```python
from build123d import *

# Parameters (mm, degrees)
EXTRUDE_1_DEPTH     = 12
SKETCH_2_R          = 8
CUT_EXTRUDE_1_DEPTH = 8
SKETCH_3_R          = 2.5
CUT_EXTRUDE_2_DEPTH = 10


with BuildPart() as part:
    # 草图1 → 凸台-拉伸1 (new body)
    with BuildSketch(Plane(origin=(0, 0, 0), x_dir=(0, 0, -1), z_dir=(1, 0, 0))):
        with BuildLine():
            Line((-27, 20), (27, 20))
            ThreePointArc((27, 20), (30.535533906, 18.535533906), (32, 15))
            Line((32, 15), (32, -15))
            ThreePointArc((32, -15), (30.535533906, -18.535533906), (27, -20))
            Line((27, -20), (-27, -20))
            ThreePointArc((-27, -20), (-30.535533906, -18.535533906), (-32, -15))
            Line((-32, -15), (-32, 15))
            ThreePointArc((-32, 15), (-30.535533906, 18.535533906), (-27, 20))
        make_face()
    extrude(amount=EXTRUDE_1_DEPTH)

    # 草图2 → 切除-拉伸1 (cut)
    with BuildSketch(Plane.ZY):
        Circle(SKETCH_2_R)
    extrude(amount=-CUT_EXTRUDE_1_DEPTH, mode=Mode.SUBTRACT)

    # 草图3 → 切除-拉伸2 (cut)
    with BuildSketch(Plane.XZ.offset(20)):
        with Locations((4, 0)):
            Circle(SKETCH_3_R)
    extrude(amount=-CUT_EXTRUDE_2_DEPTH, mode=Mode.SUBTRACT)


solid = part.part
```
Here's how the part is built. I have some questions about the finished solid (model axes, mm). A direction names the side the tool comes from. Coordinates: 2 decimals unless noted, no trailing zeros. Write each loop counter-clockwise with the first axis right and the second up, starting at its lowest first coordinate (ties: lowest second). Pieces come first, ordered by that corner, then holes. Notation, with made-up numbers: (-33.5, 64.5) -> (-15.5, 64.5) arc R16 cw to (-15.5, 80.5) -> close; hole circle Ø8 at (1, 16). An arc over 180 degrees is marked (long way). Use a Markdown table: item, result. Add a question column.
(1) If we section it at C-C, the plane z = 0: Write out the boundary of the cut face in (x, y), and give its area (3 significant figures).
(2) If we section it at B-B, the plane y = 0: Write out the boundary of the cut face in (x, z), and give its area (3 significant figures).
(3) For faces 1 (the flat face through (7, -20, 0)), 2 (the flat face through (8, 0, 0)), 3 (the cylindrical face through (6.385, -15.07, 0.751)), which set-ups out of +Z, -Z, +X, -X, +Y, -Y let a thin tool reach every point of the face, with its end or its side?
(4) I'm going to push flat-ended pins straight in: P1, Ø1.5, axis at x = 4, z = 0.5, coming from the -Y side; P2, Ø5, axis at y = 0.5, z = -0.5, coming from the -X side. Where does each tip first touch, or does it pass through?
(5) Please list where these lines run through material, in increasing order: line 1 (Y direction, x = 5.75, z = 0); line 2 (Z direction, x = 7.5, y = 1); line 3 (Z direction, x = 4, y = -18).
(6) If we section it at D-D, the plane y = -5.5: Write out the boundary of the cut face in (x, z).
(7) We'd pull the mould along X, two halves only. Please class faces 4 (the cylindrical face through (6, 19, -30)), 5 (the flat face through (12, 0, 0)), 6 (the flat face through (0, 5, -8)), 7 (the flat face through (4, -10, 0)): +X half, -X half, draft (parallel to the pull), parting line (faces both ways), or undercut.
(8) If we section it at A-A, the plane x = 4: Write out the boundary of the cut face in (y, z), and give its area (3 significant figures).
Outcome:
| question | item | result |
|---|---|---|
| 1 | outline | (0, -20) -> (1.5, -20) -> (1.5, -10) -> (6.5, -10) -> (6.5, -20) -> (12, -20) -> (12, 20) -> (0, 20) -> (0, 8) -> (8, 8) -> (8, -8) -> (0, -8) -> close |
| 1 | area | 302 mm^2 |
| 2 | outline | (0, -32) -> (12, -32) -> (12, 32) -> (0, 32) -> (0, 8) -> (8, 8) -> (8, -8) -> (0, -8) -> close |
| 2 | area | 640 mm^2 |
| 3 | face 1 | +Z, -Z, +X, -X, -Y |
| 3 | face 2 | -X |
| 3 | face 3 | -Y |
| 4 | P1 | stops at y = -10 |
| 4 | P2 | stops at x = 8 |
| 5 | line 1 | y = -10 to -8, 8 to 20 |
| 5 | line 2 | z = -32 to -7.94, 7.94 to 32 |
| 5 | line 3 | z = -31 to -2.5, 2.5 to 31 |
| 6 | outline | (0, -32) -> (12, -32) -> (12, 32) -> (0, 32) -> (0, 5.81) -> (8, 5.81) -> (8, -5.81) -> (0, -5.81) -> close |
| 7 | face 4 | draft |
| 7 | face 5 | +X half |
| 7 | face 6 | -X half |
| 7 | face 7 | undercut |
| 8 | outline | (-20, -27) arc R5 ccw to (-15, -32) -> (15, -32) arc R5 ccw to (20, -27) -> (20, 27) arc R5 ccw to (15, 32) -> (-15, 32) arc R5 ccw to (-20, 27) -> (-20, 2.5) -> (-10, 2.5) -> (-10, -2.5) -> (-20, -2.5) -> close; hole circle Ø16 at (0, 0) |
| 8 | area | 2,290 mm^2 |
